```python
from build123d import *

# Parameters (mm, degrees)
SKETCH6_R           = 16.7005
SKETCH6_R_2         = 15.875
BOSS_EXTRUDE1_DEPTH = 2.54
SKETCH7_R           = 5.588
SKETCH7_R_2         = 5.08
BOSS_EXTRUDE2_DEPTH = 2.54


with BuildPart() as part:
    # Loft1: read off the stored shape, not the designer's step
    # Loft1: loft between two sections, ruled curve by curve
    loft1_from = [
        Edge.make_bspline([(-15.531591954, 6.138106517, 0), (-3.25537892, 37.201290426, 0), (27.807804989, 24.925077391, 0), (15.531591954, -6.138106517, 0), (3.25537892, -37.201290426, 0), (-27.807804989, -24.925077391, 0), (-15.531591954, 6.138106517, 0)], [0, 0, 0, 0, 0.5, 0.5, 0.5, 1, 1, 1, 1], 3, [1, 0.333333333, 0.333333333, 1, 0.333333333, 0.333333333, 1]),
    ]
    loft1_to = [
        Edge.make_bspline([(-1.095329605, 5.479598257, -25.4), (9.863866909, 7.670257467, -25.4), (12.054526119, -3.288939047, -25.4), (1.095329605, -5.479598257, -25.4), (-9.863866909, -7.670257467, -25.4), (-12.054526119, 3.288939047, -25.4), (-1.095329605, 5.479598257, -25.4)], [0, 0, 0, 0, 0.5, 0.5, 0.5, 1, 1, 1, 1], 3, [1, 0.333333333, 0.333333333, 1, 0.333333333, 0.333333333, 1]),
    ]
    loft1 = Solid(Shell([*[Face.make_surface_from_curves(loft1_from[k], loft1_to[k]) for k in range(1)], Face(Wire(loft1_from)), Face(Wire(loft1_to))]))
    add(loft1)

    # Sketch6 → Boss-Extrude1 (add)
    with BuildSketch(Plane.XY):
        with Locations(Location((0, 0, 0), (0, 0, 158.436))):
            Circle(SKETCH6_R)
        Circle(SKETCH6_R_2, mode=Mode.SUBTRACT)
    extrude(amount=BOSS_EXTRUDE1_DEPTH)

    # Sketch7 → Boss-Extrude2 (add)
    with BuildSketch(Plane(origin=(0, 0, -25.4), x_dir=(-1, 0, 0), z_dir=(0, 0, -1))):
        with Locations(Location((0, 0, 0), (0, 0, 78.696))):
            Circle(SKETCH7_R)
        Circle(SKETCH7_R_2, mode=Mode.SUBTRACT)
    extrude(amount=BOSS_EXTRUDE2_DEPTH)


solid = part.part
```
Source: CAD feature listing. Evaluate the final solid. Frame: model axes, mm. A direction names the side the tool comes from. Give positions to 0.01 mm unless a question says otherwise; leave off trailing zeros. One line per item, written item: value. Start each with the question number.
Q1. Set-up query: faces 1 (the face through (0, 0, -25.4)), 2 (the face through (0, 0, 0)), 3 (the face through (-11.996, 11.619, 1.252)). Return all of +Z, -Z, +X, -X, +Y, -Y with unobstructed straight access to the full face (end or side cutting, diameter ignored); none if empty.
Q2. First-contact query: pin 1 Ø1.5 at (y, z) = (4.5, -8.5) entering from -X; pin 2 Ø8 at (x, y) = (-5.5, -1.5) entering from -Z; pin 3 Ø2 at (y, z) = (2, -6) entering from +X; pin 4 Ø16.5 at (x, y) = (0, 0) entering from +Z. Flat tips, straight axial feed; report the tip coordinate or a pass-through.
Q3. Material intervals for probe 1 along Y at (x, z) = (0, 1.8) (1 decimal); probe 2 along Y at (x, z) = (0, -26); probe 3 along Z at (x, y) = (0, 1.5), sorted ascending. Write a range as from..to.
Answer:
1. face 1: -Z
1. face 2: +Z
1. face 3: +Z, -Z
2. pin 1: stops at x = -11.86
2. pin 2: stops at z = -27.94
2. pin 3: stops at x = 13.91
2. pin 4: stops at z = 0
3. probe 1: y = -16.7..-15.9, 15.9..16.7
3. probe 2: y = -5.59..-5.08, 5.08..5.59
3. probe 3: z = -25.4..0
